from build123d import *

# Parameters (mm, degrees)
F0_W          = 9.14383
F0_H          = 9.140982
F1_DEPTH      = 5.588
F1_DEPTH_BACK = 5.588
F2_T          = -0.762
F3_R          = 2.280613
F4_DEPTH      = 0.762
F5_R          = 2.282355
F6_DEPTH      = 0.762


with BuildPart() as f1:
    # F0 (on Front) → F1 (new body, two sides)
    with BuildSketch(Plane.XZ) as f1_sk:
        Rectangle(F0_W, F0_H)
    extrude(amount=F1_DEPTH)
    extrude(f1_sk.sketch, amount=-F1_DEPTH_BACK)

    # F2
    f2_openings = [f1.faces().sort_by_distance(p)[0] for p in [
        (0, 0, 4.570491),
        (4.571915, 0, 0),
        (0, -5.588, 0),
        (0, 5.588, 0),
    ]]
    offset(amount=F2_T, openings=f2_openings)

    # F3 (on face) → F4 (cut)
    with BuildSketch(Plane.YZ.offset(-3.809915)):
        with Locations((0, 0.381)):
            Circle(F3_R)
    extrude(amount=-F4_DEPTH, mode=Mode.SUBTRACT)

    # F5 (on face) → F6 (cut)
    with BuildSketch(Plane.XY.offset(-3.808491)):
        with Locations((0.381, 0)):
            Circle(F5_R)
    extrude(amount=-F6_DEPTH, mode=Mode.SUBTRACT)


solid = f1.part
Design review of the part built by this model. Coordinates are the model's own, in mm. A direction names the side the tool comes from. Round coordinates to 2 decimals unless told otherwise and drop trailing zeros. Write each loop counter-clockwise with the first axis right and the second up, starting at its lowest first coordinate (ties: lowest second). Pieces come first, ordered by that corner, then holes. Notation, with made-up numbers: (28, 87.5) -> (81, 87.5) arc R14 ccw to (81, 109.5) -> close; hole circle Ø9 at (5.25, -16). An arc over 180 degrees is marked (long way). One line per item, written item: value. Start each with the question number.
Q1. Insertion check: P1, Ø2, axis at x = 0.5, y = 2, coming from the +Z side. The pin has a flat end and moves straight along its axis. Give the tip position at first contact, or say it passes through.
Q2. Add section D-D (y = 4.5). Give the boundary of the cut face in (x, z), then the cut area to 3 significant figures.
Q3. Add section B-B (x = 1.5). Give the boundary of the cut face in (y, z).
Q4. To check wall thickness, follow probe 1 along Z at (x, y) = (-4.15, 0); probe 2 along Z at (x, y) = (2, -3); probe 3 along Y at (x, z) = (-4, 0). State the ranges of each line that lie inside material, in increasing order.
Q5. The part is to be moulded in two halves that separate along Y. For faces 1 (the face through (-2.1, -0.1, -4.57)), 2 (the face through (-0.11, -2.23, -4.18)), 3 (the face through (-4, 5.588, -2)), 4 (the face through (-4.19, -0.3, 2.64)), say which applies: pulls with the +Y half, pulls with the -Y half, needs draft (parallel to the pull), parting line crosses it, or undercut.
Q6. Add section C-C (z = 4.25). Give the boundary of the cut face in (x, y).
Q7. Tool access review of faces 5 (the face through (-4, -5.588, -2)), 6 (the face through (-2, -1, -3.808)): name each direction out of +Z, -Z, +X, -X, +Y, -Y from which nothing blocks a thin tool from reaching the whole face with its end or side.
Q8. Add section A-A (y = 0). Give the boundary of the cut face in (x, z).
Response:
1. P1: stops at z = -3.81
2. outline: (-4.57, -4.57) -> (4.57, -4.57) -> (4.57, -3.81) -> (-3.81, -3.81) -> (-3.81, 4.57) -> (-4.57, 4.57) -> close
2. area: 13.4 mm^2
3. outline: (-5.59, -4.57) -> (-1.99, -4.57) -> (-1.99, -3.81) -> (-5.59, -3.81) -> close; (1.99, -4.57) -> (5.59, -4.57) -> (5.59, -3.81) -> (1.99, -3.81) -> close
4. probe 1: z = -4.57 to -1.9, 2.66 to 4.57
4. probe 2: z = -4.57 to -3.81
4. probe 3: y = -5.59 to -2.25, 2.25 to 5.59
5. face 1: needs draft
5. face 2: undercut
5. face 3: pulls with the +Y half
5. face 4: undercut
6. outline: (-4.57, -5.59) -> (-3.81, -5.59) -> (-3.81, 5.59) -> (-4.57, 5.59) -> close
7. face 5: +Z, -Z, +X, -X, -Y
7. face 6: +Z, +X, +Y, -Y
8. outline: (-4.57, -4.57) -> (-1.9, -4.57) -> (-1.9, -3.81) -> (-3.81, -3.81) -> (-3.81, -1.9) -> (-4.57, -1.9) -> close; (-4.57, 2.66) -> (-3.81, 2.66) -> (-3.81, 4.57) -> (-4.57, 4.57) -> close; (2.66, -4.57) -> (4.57, -4.57) -> (4.57, -3.81) -> (2.66, -3.81) -> close
